Part model, mm, in its own coordinate system. Coordinates: 2 decimals unless noted, no trailing zeros. One line per question, with ' | ' between items. Start each with the question number.
Item 1: Pin check, flat tips, straight feed: pin 1 (3 mm diameter, centred on x = -2.5, y = -272, fed in from -Z); pin 2 (1 mm diameter, centred on x = -1, z = -3.5, fed in from +Y); pin 3 (5 mm diameter, centred on x = 0, z = -6.05, fed in from +Y). Stop position of each tip, or through.
Item 2: Two-plate mould, pull along X, no slides. Class faces 1 (the flat face through (8, -272, -1)), 2 (the flat face through (-8, -272, -1)), 3 (the flat face through (-0.112, -270.012, -11.797)), 4 (the cylindrical face through (-2.05, -271.04, -6.51)): pulls with the +X half, pulls with the -X half, needs draft (parallel to the pull), parting line crosses it, or undercut.
Item 3: Probe probe 1 along Y at (x, z) = (-5.5, -7.5); probe 2 along Y at (x, z) = (4.5, 1); probe 3 along X at (y, z) = (-268.5, -7.75). List the from-to ranges inside material, lowest first. Write a range as [from, to].
from build123d import *

# Parameters (mm, degrees)
SKETCH8_R          = 2.1
CUT_EXTRUDE2_DEPTH = 20.175814847


with BuildPart() as part:
    # Sweep1: sweep along a path in Sketch5
    with BuildLine() as sweep1_path:  # in the path sketch's own coordinates; laid on its plane below (add() does not lay a ready-made edge on the line's plane)
        add(Edge.make_bspline(
            [(12, -273.587448275), (1.118694171, -276.48109121), (-10, -278.234045614)],
            knots=[0, 0, 0, 1, 1, 1], degree=2))
    # Sketch2 → Sweep1 (sweep)
    with BuildSketch(Plane.XY):
        with BuildLine():
            Line((7.999671005, -275.908898325), (7.999671005, -268.48657561))
            Line((7.999671005, -268.48657561), (-8.000328995, -268.48657561))
            Line((-8.000328995, -268.48657561), (-8.000328995, -275.908898325))
            add(Edge.make_bspline(
                [(7.999671005, -275.908898325), (-0.000325582, -277.064252884), (-8.000328995, -275.908898325)],
                knots=[0, 0, 0, 1, 1, 1], degree=2))
        make_face()
    sweep(path=Plane(origin=(0, 0, 0), x_dir=(0, 0, -1), z_dir=(1, 0, 0)) * sweep1_path.line)

    # Sketch8 → Cut-Extrude2 (cut, through all)
    with BuildSketch(Plane(origin=(0, -265.669886224, 0), x_dir=(1, 0, 0), z_dir=(0, 1, 0))):
        with Locations(Location((-4.6e-08, 6.050192376, 0), (0, 0, 270))):
            Circle(SKETCH8_R)
    extrude(amount=-CUT_EXTRUDE2_DEPTH, mode=Mode.SUBTRACT)


solid = part.part
From the geometry:
1) pin 1: z = -12 | pin 2: y = -267.59 | pin 3: y = -266.47
2) face 1: pulls with the +X half | face 2: pulls with the -X half | face 3: needs draft | face 4: undercut
3) probe 1: [-274.53, -266.74] | probe 2: [-276.51, -268.7] | probe 3: [-8, -1.23], [1.23, 8]
